from build123d import *

# Parameters (mm, degrees)
F1_DEPTH = 1000


with BuildPart() as f1:
    # F0 (on Top) → F1 (new body)
    with BuildSketch(Plane.XY):
        with BuildLine():
            Line((0, 355), (0, 0))
            Line((0, 0), (107.5, 0))
            Line((107.5, 0), (107.5, 12))
            ThreePointArc((107.5, 12), (136.911107, 23.510225), (148.804216, 52.7686))
            Line((148.804216, 52.7686), (160.804216, 52.7686))
            Line((160.804216, 52.7686), (160.804216, 62.7686))
            Line((160.804216, 62.7686), (198.804216, 62.7686))
            ThreePointArc((198.804216, 62.7686), (206.045742, 59.934201), (209.066943, 52.7686))
            Line((209.066943, 52.7686), (229.066943, 52.771947))
            Line((229.066943, 52.771947), (229.066943, 133.853948))
            Line((229.066943, 133.853948), (241.066943, 133.853948))
            Line((241.066943, 133.853948), (241.066943, 146.052128))
            ThreePointArc((241.066943, 146.052128), (265.815681, 156.303391), (276.066943, 181.052128))
            Line((276.066943, 181.052128), (288.066943, 181.052128))
            Line((288.066943, 181.052128), (288.066943, 193.052128))
            ThreePointArc((288.066943, 193.052128), (326.957816, 209.161255), (343.066943, 248.052128))
            ThreePointArc((343.066943, 248.052128), (356.657186, 284.249256), (390.711745, 302.558101))
            Line((390.711745, 302.558101), (390.711745, 337.558101))
            Line((390.711745, 337.558101), (107.5, 355))
            Line((107.5, 355), (0, 355))
        make_face()
    extrude(amount=F1_DEPTH)


solid = f1.part
Geometry: final body of the model. Coordinates: model frame, mm. A direction names the side the tool comes from. Coordinates: 2 decimals unless noted, no trailing zeros. Loops run counter-clockwise (first coordinate to the right, second up) from the corner with the lowest first, then second, coordinate; pieces in that order, holes last. Notation, with made-up numbers: M 80,-27 L 85,-27 A10 ccw 85,-23 Z; hole C 74.5,84 d5. An arc over 180 degrees is marked long. One line per item, written item: value. Start each with the question number.
1) Reachability of faces 1 (the flat face through (251.088, 346.157, 493)), 2 (the flat face through (229.067, 93, 493)) from +Z, -Z, +X, -X, +Y, -Y: full face, straight path, thin tool, end or side. Return the list, or none.
2) Cut plane C-C (y = 161). Return loops of the section in (x, z), then the cut area to 3 significant figures.
3) Cut plane B-B (y = 96.5). Return loops of the section in (x, z).
4) Material intervals for L1, parallel to X at y = 190.5, z = 305.5; L2, parallel to X at y = 45.5, z = 647.5; L3, parallel to Y at x = 245.5, z = 127, sorted ascending. Write a range as from..to.
5) Draft query along X for faces 3 (the flat face through (390.712, 320, 493)), 4 (the flat face through (55, 355, 493)), 5 (the flat face through (180, 62.769, 493)). Return one class per face: released by +X, released by -X, zero draft, split by the parting line, or undercut.
6) Cut plane A-A (z = 638.5). Return loops of the section in (x, y), then the cut area to 3 significant figures.
7) Pin query (flat end, axial travel): P1, Ø2, axis at x = 159, z = 273.5, coming from the +Y side; P2, Ø8, axis at x = 307, z = 685.5, coming from the +Y side; P3, Ø9.5, axis at x = 283, z = 455, coming from the -Y side. Return the tip coordinate at first contact, or that it passes through.
Evaluation:
1. face 1: +Z, -Z, +X, +Y
1. face 2: +Z, -Z, +X, -Y
2. outline: M 0,0 L 269.75,0 L 269.75,1000 L 0,1000 Z
2. area: 270,000 mm^2
3. outline: M 0,0 L 229.07,0 L 229.07,1000 L 0,1000 Z
4. L1: 0..288.07
4. L2: 0..148.28
4. L3: 146.33..346.5
5. face 3: released by +X
5. face 4: zero draft
5. face 5: undercut
6. outline: M 0,0 L 107.5,0 L 107.5,12 A40 ccw 148.8,52.77 L 160.8,52.77 L 160.8,62.77 L 198.8,62.77 A10 cw 209.07,52.77 L 229.07,52.77 L 229.07,133.85 L 241.07,133.85 L 241.07,146.05 A35 ccw 276.07,181.05 L 288.07,181.05 L 288.07,193.05 A55 ccw 343.07,248.05 A55 cw 390.71,302.56 L 390.71,337.56 L 107.5,355 L 0,355 Z
6. area: 96,500 mm^2
7. P1: y = 351.89
7. P2: y = 342.96
7. P3: y = 181.05
